```python
from build123d import *

# Parameters (mm, degrees)
SKETCH1_R                       = 7.14375
BOSS_EXTRUDE1_DEPTH             = 12.7
SKETCH3_R                       = 5.715
BOSS_EXTRUDE2_DEPTH             = 1.5875
F_1_4_0_25_DIAMETER_HOLE1_D     = 6.35
F_1_4_0_25_DIAMETER_HOLE1_DEPTH = 11.1125
F_1_4_0_25_DIAMETER_HOLE1_TIP   = 1.907732465


with BuildPart() as part:
    # Sketch1 → Boss-Extrude1 (new body)
    with BuildSketch(Plane(origin=(0, 0, 0), x_dir=(1, 0, 0), z_dir=(0, 1, 0))):
        with Locations(Location((0, 0, 0), (0, 0, 270))):
            Circle(SKETCH1_R)
    extrude(amount=BOSS_EXTRUDE1_DEPTH)

    # Sketch3 → Boss-Extrude2 (add)
    with BuildSketch(Plane(origin=(0, 12.7, 0), x_dir=(1, 0, 0), z_dir=(0, 1, 0))):
        with Locations(Location((0, 0, 0), (0, 0, 270))):
            Circle(SKETCH3_R)
    extrude(amount=BOSS_EXTRUDE2_DEPTH)

    # 1/4 (0.25) Diameter Hole1
    with Locations(Plane(origin=(0, 0, 0), x_dir=(-1, 0, 0), z_dir=(0, -1, 0))):
        with Locations((0, 0)):
            Hole(F_1_4_0_25_DIAMETER_HOLE1_D / 2, depth=F_1_4_0_25_DIAMETER_HOLE1_DEPTH)
            with Locations((0, 0, -(F_1_4_0_25_DIAMETER_HOLE1_DEPTH + F_1_4_0_25_DIAMETER_HOLE1_TIP / 2))):  # 118° drill point
                Cone(0, F_1_4_0_25_DIAMETER_HOLE1_D / 2, F_1_4_0_25_DIAMETER_HOLE1_TIP, mode=Mode.SUBTRACT)


solid = part.part
```
Here's how the part is built. I have some questions about the finished solid (model axes, mm). A direction names the side the tool comes from. Coordinates: 2 decimals unless noted, no trailing zeros. Loops run counter-clockwise (first coordinate to the right, second up) from the corner with the lowest first, then second, coordinate; pieces in that order, holes last. Notation, with made-up numbers: (31, 62.25) - (75, 62.25) arc R12 cw to (75, 74.25) - close; hole circle Ø7 at (-34.5, 44.25). An arc over 180 degrees is marked (long way). Return JSON: item names as keys, results as strings. Group by question number.
Item 1: If we section it at B-B on z = 3.5: Write out the boundary of the cut face in (x, y).
Item 2: We'd pull the mould along X, two halves only. Please class faces 3 (the face through (-0.69, 5.63, 3.1)), 4 (the face through (-1.5, 0, 3.1)), 5 (the face through (5.666, 13.483, -0.744)): +X half, -X half, draft (parallel to the pull), parting line (faces both ways), or undercut.
Item 3: If we section it at C-C on x = -6: Write out the boundary of the cut face in (y, z), and give its area (3 significant figures).
Item 4: I need wall thicknesses on line 1 (Z direction, x = 1.5, y = 3.25); line 2 (X direction, y = 10.25, z = -0.25); line 3 (X direction, y = 10.25, z = -0.5). Which ranges of each line are inside material? Lowest first, please. Write a range as from..to.
Item 5: On a 3-axis mill with a long thin cutter (end or side, diameter ignored), from which of +Z, -Z, +X, -X, +Y, -Y can I reach the whole of each face in a straight line? I mean faces 1 (the face through (0.12, 12.69, 0.54)), 2 (the face through (6, 12.7, 0)). Say none if no direction works.
Item 6: Will these pins go through, and if not, where does the flat tip stop? P1, Ø5.5, axis at x = 0, z = 0, coming from the -Y side; P2, Ø5, axis at x = -3, y = 5.5, coming from the +Z side; P3, Ø1, axis at x = 5.5, y = 8, coming from the -Z side.
Item 7: If we section it at D-D on y = 13.25: Write out the boundary of the cut face in (x, z) (3 decimals).
Calculated:
{
 "1": {"outline": "(-6.23, 0) - (6.23, 0) - (6.23, 12.7) - (4.52, 12.7) - (4.52, 14.29) - (-4.52, 14.29) - (-4.52, 12.7) - (-6.23, 12.7) - close"},
 "2": {"face 3": "undercut", "face 4": "draft", "face 5": "parting line"},
 "3": {"outline": "(0, -3.88) - (12.7, -3.88) - (12.7, 3.88) - (0, 3.88) - close", "area": "98.5 mm^2"},
 "4": {"line 1": "z = -6.98..-2.8, 2.8..6.98", "line 2": "x = -7.14..-3.17, 3.17..7.14", "line 3": "x = -7.13..-3.14, 3.14..7.13"},
 "5": {"face 1": "-Y", "face 2": "+Y"},
 "6": {"P1": "stops at y = 11.37", "P2": "stops at z = 7.13", "P3": "stops at z = -5.1"},
 "7": {"outline": "circle Ø11.43 at (0, 0)"}
}
